```python
from build123d import *

# Parameters (mm, degrees)
F0_W     = 101.6
F0_H     = 101.6
F2_DEPTH = 117.094
F3_DEPTH = 117.094
F4_W     = 88.9
F4_H     = 101.6
F5_DEPTH = 104.394


with BuildPart() as f2:
    # F0 (on Front) → F2 (new body)
    with BuildSketch(Plane.XZ):
        with Locations((50.8, 50.8)):
            Rectangle(F0_W, F0_H)
    extrude(amount=-F2_DEPTH)

    # F1 (on face) → F3 (cut)
    with BuildSketch(Plane.XZ):
        with BuildLine():
            Line((34.425654, 0), (59.831641, 0))
            ThreePointArc((59.831641, 0), (47.128648, 12.702994), (34.425654, 0))
        make_face()
    extrude(amount=-F3_DEPTH, mode=Mode.SUBTRACT)

    # F4 (on face) → F5 (cut)
    with BuildSketch(Plane.XY.offset(101.6)):
        with Locations((50.05706, 59.151817)):
            Rectangle(F4_W, F4_H)
    extrude(amount=-F5_DEPTH, mode=Mode.SUBTRACT)


solid = f2.part
```
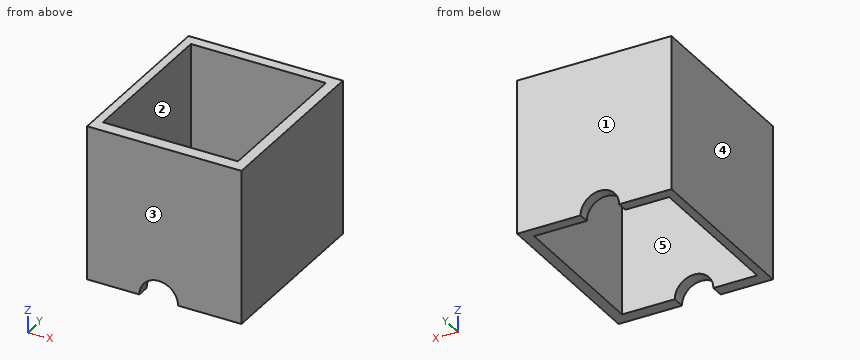
Geometry check sheet. Reference: the model listing, model coordinates, mm. Face numbers are marked on the shaded views. A direction names the side the tool comes from. Give positions to 0.01 mm unless a question says otherwise; leave off trailing zeros. Order: outer loops, then holes, each group sorted by start corner. A loop starts at its lowest first (then second) coordinate and runs counter-clockwise, first axis right, second up.
1. Access from +Z, -Z, +X, -X, +Y, -Y to the whole of each face (thin tool, end or side, straight path). Record for the marked faces 1 and 2.
2. Section check C-C, the plane x = 17. Enter the section's corners in (y, z), and give its area (3 significant figures).
3. Release check for a two-part mould opening along X. For the marked faces 3, 4 and 5 record: pulls with the +X half, pulls with the -X half, needs draft (parallel to the pull), parting line crosses it, or undercut.
4. Section check B-B, the plane z = 71.5. Enter the section's corners in (x, y), and give its area (3 significant figures).
5. Section check A-A, the plane y = 24. Enter the section's corners in (x, z).
6. Thickness scan on L1, parallel to Y at x = 88, z = 44.5; L2, parallel to X at y = 87, z = 29.5. Record the ranges inside material, lowest first.
Values follow:
1. face 1: +Z, -Z, +X, -X, +Y
1. face 2: +Z, -Z
2. outline: (0, 0) - (8.35, 0) - (8.35, 101.6) - (0, 101.6) - close; (109.95, 0) - (117.09, 0) - (117.09, 101.6) - (109.95, 101.6) - close
2. area: 1,570 mm2
3. face 3: needs draft
3. face 4: pulls with the -X half
3. face 5: undercut
4. outline: (0, 0) - (101.6, 0) - (101.6, 117.09) - (0, 117.09) - close; hole (5.61, 8.35) - (94.51, 8.35) - (94.51, 109.95) - (5.61, 109.95) - close
4. area: 2,860 mm2
5. outline: (0, 0) - (5.61, 0) - (5.61, 101.6) - (0, 101.6) - close; (94.51, 0) - (101.6, 0) - (101.6, 101.6) - (94.51, 101.6) - close
6. L1: y = 0 to 8.35, 109.95 to 117.09
6. L2: x = 0 to 5.61, 94.51 to 101.6
